Check sheet for the modelled part. Datum: model origin and axes. Units: mm. Face numbers are marked on the shaded views. A direction names the side the tool comes from. Round coordinates to 2 decimals unless told otherwise and drop trailing zeros. Loops run counter-clockwise (first coordinate to the right, second up) from the corner with the lowest first, then second, coordinate; pieces in that order, holes last. Notation, with made-up numbers: (-29.5, 64) -> (-16.5, 64) arc R22 ccw to (-16.5, 93) -> close; hole circle Ø1 at (7.5, 21.25). An arc over 180 degrees is marked (long way). Return JSON: item names as keys, results as strings.
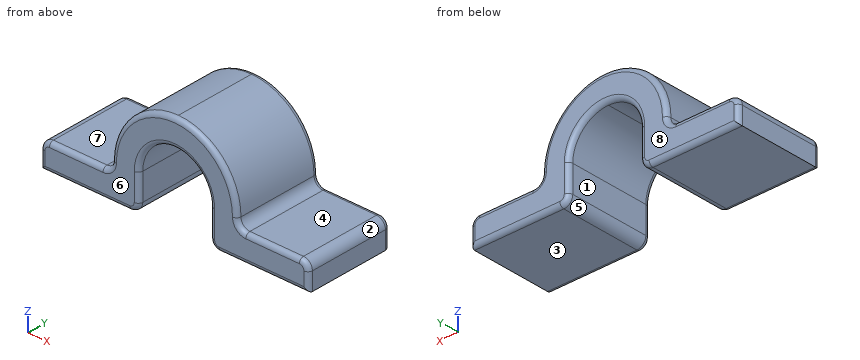
from build123d import *

# Parameters (mm, degrees)
F1_DEPTH     = 10
F2_R         = 0.99999
F3_T1_DEPTH  = 1e-05
F3_T3_DEPTH  = 3.00001
F3_T5_DEPTH  = 11.25001
F3_T7_DEPTH  = 6.00002
F3_T9_DEPTH  = 3.25001
F3_T12_ANGLE = 107.9121236547
F3_T14_ANGLE = 100.2354992312
F3_T16_ANGLE = 90
F3_T18_ANGLE = 107.9121236547
F3_T20_ANGLE = 90
F3_T22_ANGLE = 100.2354992312
F3_T24_ANGLE = 90
F3_T26_ANGLE = 90
F3_T28_ANGLE = 90
F3_T30_ANGLE = 90


# Not quite as in the source:
# - a fillet or chamfer that OpenCascade refuses, or shapes differently, is made with other operations: its cross-section is extruded or revolved along the edge and cut away or added
# - a fillet or chamfer is up to 0.001 mm smaller than in the source, because OpenCascade refuses the exact size


with BuildPart() as f1:
    # F0 (on Front) → F1 (new body)
    with BuildSketch(Plane.XZ):
        with BuildLine():
            Line((7, 3), (7, 4))
            ThreePointArc((7, 4), (6.6787700412, 1.9038056538), (5.7445626465, 0))
            Line((5.7445626465, 0), (7, 0))
            Line((7, 0), (15, 0))
            Line((15, 0), (15, 3))
            Line((15, 3), (7, 3))
        make_face()
        with BuildLine():
            Line((7, 4), (4, 4))
            Line((4, 4), (4, 0))
            Line((4, 0), (5.7445626465, 0))
            ThreePointArc((5.7445626465, 0), (6.6787700412, 1.9038056538), (7, 4))
        make_face()
        with BuildLine():
            Line((0, 11), (0, 8))
            ThreePointArc((0, 8), (2.8284271247, 6.8284271247), (4, 4))
            Line((4, 4), (7, 4))
            ThreePointArc((7, 4), (4.9497474683, 8.9497474683), (0, 11))
        make_face()
    extrude(amount=F1_DEPTH)

    # F2 (radius 1 in the source; OpenCascade refuses exactly that, so slightly less here)
    f2_edges = [f1.edges().sort_by_distance(p)[0] for p in [
        (7, -5, 3),
        (4, -5, 0),
        (15, -5, 3),
    ]]
    fillet(f2_edges, radius=F2_R)

    # F3: fillet of radius 0.5 on 5 edges, made by hand

    # F3_s2 → F3_t1 (cut)
    with BuildSketch(Plane.XY.offset(3.99999)):
        with BuildLine():
            ThreePointArc((6.5, -10), (6.8535533906, -9.8535533906), (7, -9.5))
            Line((7, -9.5), (7, -10))
            Line((7, -10), (6.5, -10))
        make_face()
        with BuildLine():
            ThreePointArc((6.5, 0), (6.8535533906, -0.1464466094), (7, -0.5))
            Line((7, -0.5), (7, 0))
            Line((7, 0), (6.5, 0))
        make_face()
    extrude(amount=F3_T1_DEPTH, mode=Mode.SUBTRACT)

    # F3_s4 → F3_t3 (cut)
    with BuildSketch(Plane.XY.offset(0.99999)):
        with BuildLine():
            ThreePointArc((4.5, 0), (4.1464466094, -0.1464466094), (4, -0.5))
            Line((4, -0.5), (4, 0))
            Line((4, 0), (4.5, 0))
        make_face()
        with BuildLine():
            ThreePointArc((4.5, -10), (4.1464466094, -9.8535533906), (4, -9.5))
            Line((4, -9.5), (4, -10))
            Line((4, -10), (4.5, -10))
        make_face()
    extrude(amount=F3_T3_DEPTH, mode=Mode.SUBTRACT)

    # F3_s6 → F3_t5 (cut)
    with BuildSketch(Plane.YZ.offset(4.99999)):
        with BuildLine():
            ThreePointArc((0, 0.5), (-0.1464466094, 0.1464466094), (-0.5, 0))
            Line((-0.5, 0), (0, 0))
            Line((0, 0), (0, 0.5))
        make_face()
        with BuildLine():
            ThreePointArc((-9.5, 0), (-9.8535533906, 0.1464466094), (-10, 0.5))
            Line((-10, 0.5), (-10, 0))
            Line((-10, 0), (-9.5, 0))
        make_face()
    extrude(amount=F3_T5_DEPTH, mode=Mode.SUBTRACT)

    # F3_s8 → F3_t7 (cut)
    with BuildSketch(Plane.YZ.offset(7.99999)):
        with BuildLine():
            ThreePointArc((0, 2.5), (-0.1464466094, 2.8535533906), (-0.5, 3))
            Line((-0.5, 3), (0, 3))
            Line((0, 3), (0, 2.5))
        make_face()
        with BuildLine():
            ThreePointArc((-10, 2.5), (-9.8535533906, 2.8535533906), (-9.5, 3))
            Line((-9.5, 3), (-10, 3))
            Line((-10, 3), (-10, 2.5))
        make_face()
    extrude(amount=F3_T7_DEPTH, mode=Mode.SUBTRACT)

    # F3_s10 → F3_t9 (cut)
    with BuildSketch(Plane.XY.offset(-1.25)):
        with BuildLine():
            ThreePointArc((15, -0.5), (14.8535533906, -0.1464466094), (14.5, 0))
            Line((14.5, 0), (15, 0))
            Line((15, 0), (15, -0.5))
        make_face()
        with BuildLine():
            ThreePointArc((15, -9.5), (14.8535533906, -9.8535533906), (14.5, -10))
            Line((14.5, -10), (15, -10))
            Line((15, -10), (15, -9.5))
        make_face()
    extrude(amount=F3_T9_DEPTH, mode=Mode.SUBTRACT)

    # F3_s11 → F3_t12 (revolve, cut)
    with BuildSketch(Plane(origin=(1.1706017221, 0, 0.37836761), x_dir=(0, 1, 0), z_dir=(-0.9515293466, 0, -0.3075579661))):
        with BuildLine():
            ThreePointArc((-10, -8.3061173865), (-9.8535533906, -7.9525639959), (-9.5, -7.8061173865))
            Line((-9.5, -7.8061173865), (-10, -7.8061173865))
            Line((-10, -7.8061173865), (-10, -8.3061173865))
        make_face()
    revolve(axis=Axis((0, -10, 4), (0, 1, 0)), revolution_arc=F3_T12_ANGLE, mode=Mode.SUBTRACT)

    # F3_s13 → F3_t14 (revolve, cut)
    with BuildSketch(Plane.XY.offset(4)):
        with BuildLine():
            ThreePointArc((6.5, -10), (6.8535533906, -9.8535533906), (7, -9.5))
            Line((7, -9.5), (7, -10))
            Line((7, -10), (6.5, -10))
        make_face()
    revolve(axis=Axis((0, -10, 4), (0, -1, 0)), revolution_arc=F3_T14_ANGLE, mode=Mode.SUBTRACT)

    # F3_s15 → F3_t16 (revolve, cut)
    with BuildSketch(Plane.YZ.offset(7.99999)):
        with BuildLine():
            ThreePointArc((0, 2.5), (-0.1464466094, 2.8535533906), (-0.5, 3))
            Line((-0.5, 3), (0, 3))
            Line((0, 3), (0, 2.5))
        make_face()
    revolve(axis=Axis((7.99999, 0, 3.99999), (0, 1, 0)), revolution_arc=F3_T16_ANGLE, mode=Mode.SUBTRACT)

    # F3_s17 → F3_t18 (revolve, cut)
    with BuildSketch(Plane(origin=(1.1706017221, 0, 0.37836761), x_dir=(0, 1, 0), z_dir=(-0.9515293466, 0, -0.3075579661))):
        with BuildLine():
            ThreePointArc((0, -8.3061173865), (-0.1464466094, -7.9525639959), (-0.5, -7.8061173865))
            Line((-0.5, -7.8061173865), (0, -7.8061173865))
            Line((0, -7.8061173865), (0, -8.3061173865))
        make_face()
    revolve(axis=Axis((0, 0, 4), (0, 1, 0)), revolution_arc=F3_T18_ANGLE, mode=Mode.SUBTRACT)

    # F3_s19 → F3_t20 (revolve, cut)
    with BuildSketch(Plane.XY.offset(0.99999)):
        with BuildLine():
            ThreePointArc((4.5, 0), (4.1464466094, -0.1464466094), (4, -0.5))
            Line((4, -0.5), (4, 0))
            Line((4, 0), (4.5, 0))
        make_face()
    revolve(axis=Axis((4.99999, 0, 0.99999), (0, -1, 0)), revolution_arc=F3_T20_ANGLE, mode=Mode.SUBTRACT)

    # F3_s21 → F3_t22 (revolve, cut)
    with BuildSketch(Plane.XY.offset(4)):
        with BuildLine():
            ThreePointArc((6.5, 0), (6.8535533906, -0.1464466094), (7, -0.5))
            Line((7, -0.5), (7, 0))
            Line((7, 0), (6.5, 0))
        make_face()
    revolve(axis=Axis((0, 0, 4), (0, -1, 0)), revolution_arc=F3_T22_ANGLE, mode=Mode.SUBTRACT)

    # F3_s23 → F3_t24 (revolve, cut)
    with BuildSketch(Plane.XY.offset(2.00001)):
        with BuildLine():
            ThreePointArc((14.5, 0), (14.8535533906, -0.1464466094), (15, -0.5))
            Line((15, -0.5), (15, 0))
            Line((15, 0), (14.5, 0))
        make_face()
    revolve(axis=Axis((14.00001, 0, 2.00001), (0, -1, 0)), revolution_arc=F3_T24_ANGLE, mode=Mode.SUBTRACT)

    # F3_s25 → F3_t26 (revolve, cut)
    with BuildSketch(Plane.YZ.offset(7.99999)):
        with BuildLine():
            ThreePointArc((-10, 2.5), (-9.8535533906, 2.8535533906), (-9.5, 3))
            Line((-9.5, 3), (-10, 3))
            Line((-10, 3), (-10, 2.5))
        make_face()
    revolve(axis=Axis((7.99999, -10, 3.99999), (0, 1, 0)), revolution_arc=F3_T26_ANGLE, mode=Mode.SUBTRACT)

    # F3_s27 → F3_t28 (revolve, cut)
    with BuildSketch(Plane.XY.offset(2.00001)):
        with BuildLine():
            ThreePointArc((15, -9.5), (14.8535533906, -9.8535533906), (14.5, -10))
            Line((14.5, -10), (15, -10))
            Line((15, -10), (15, -9.5))
        make_face()
    revolve(axis=Axis((14.00001, -10, 2.00001), (0, -1, 0)), revolution_arc=F3_T28_ANGLE, mode=Mode.SUBTRACT)

    # F3_s29 → F3_t30 (revolve, cut)
    with BuildSketch(Plane.XY.offset(0.99999)):
        with BuildLine():
            ThreePointArc((4.5, -10), (4.1464466094, -9.8535533906), (4, -9.5))
            Line((4, -9.5), (4, -10))
            Line((4, -10), (4.5, -10))
        make_face()
    revolve(axis=Axis((4.99999, -10, 0.99999), (0, -1, 0)), revolution_arc=F3_T30_ANGLE, mode=Mode.SUBTRACT)

    # F4: F1 across face


with BuildPart() as f1_1:
    add(f1.part)
    add(f1.part.mirror(Plane(origin=(0, -5, 9.5), x_dir=(0, -1, 0), z_dir=(-1, 0, 0))))


solid = f1_1.part
Q1. Tool access check on the marked faces 4, 5, 6, 7 and 8. Record the directions out of +Z, -Z, +X, -X, +Y, -Y that give a thin tool (end or side, any length) a straight path to the whole face; none if there is none.
Results list:
{"face 4": "+Z, +X, +Y, -Y", "face 5": "-Z, +Y, -Y", "face 6": "+Z, -Z, +X, -X, -Y", "face 7": "+Z, -X, +Y, -Y", "face 8": "+Z, -Z, +X, -X, +Y"}
Q2. Material ranges on line 1 (X direction, y = -8.5, z = 3.25); line 2 (X direction, y = -5.75, z = 6); line 3 (Z direction, x = -8.25, y = -1), recorded low to high.
Results list:
{"line 1": "-7.34 to -4, 4 to 7.34", "line 2": "-6.71 to -3.46, 3.46 to 6.71", "line 3": "0 to 3"}
Q3. Go/stop test with flat-tipped pins: pin 1 (3 mm diameter, centred on y = -3, z = 8, fed in from +X); pin 2 (5 mm diameter, centred on y = -7.5, z = 2.5, fed in from -X); pin 3 (3 mm diameter, centred on x = 12.5, y = -3.5, fed in from +Z). Record where each tip stops, or that it passes through.
Results list:
{"pin 1": "x = 6.54", "pin 2": "x = -15", "pin 3": "z = 3"}
Q4. Draft check along X on the marked faces 1, 2 and 3. Enter one of: released by +X, released by -X, zero draft, split by the parting line, or undercut.
Results list:
{"face 1": "undercut", "face 2": "released by +X", "face 3": "zero draft"}
Q5. Section check A-A (x = 12.5). Record the boundary of the cut face in (y, z), then the cut area to 3 significant figures.
Results list:
{"outline": "(-10, 0.5) arc R0.5 ccw to (-9.5, 0) -> (-0.5, 0) arc R0.5 ccw to (0, 0.5) -> (0, 2.5) arc R0.5 ccw to (-0.5, 3) -> (-9.5, 3) arc R0.5 ccw to (-10, 2.5) -> close", "area": "29.8 mm^2"}
